Read the model definition and answer for the solid it produces. Units are mm, in the model's axes. A direction names the side the tool comes from. Round coordinates to 2 decimals unless told otherwise and drop trailing zeros. Order: outer loops, then holes, each group sorted by start corner. A loop starts at its lowest first (then second) coordinate and runs counter-clockwise, first axis right, second up. Notation, with made-up numbers: (49.25, 43.5) -> (105.25, 43.5) arc R22 cw to (105.25, 69.5) -> close; hole circle Ø10 at (-8, 77). An arc over 180 degrees is marked (long way). Use a Markdown table: item, result. Add a question column.
1. Section B-B, the plane y = -12.5 is taken. Give the number of separate pieces and of enclosed holes in the cut face, then the cut area to 3 significant figures.
2. For faces 5 (the face through (165.216, -15, -110)), 6 (the face through (-25, -20, -110)), 7 (the face through (100, -15, 265)), 8 (the face through (-4, 0, -4)), determine the directions among +Z, -Z, +X, -X, +Y, -Y from which every point of the face is accessible in a straight line to the end or side of a thin tool.
3. Section A-A, the plane z = 16.5 is taken. Give the vertices of the cut face in (x, y).
4. The mould has two halves that part along X. Classify faces 1 (the face through (-4, -30, -4)), 2 (the face through (-110, -15, -110)), 3 (the face through (-282.89, -14.79, 281.96)), 4 (the face through (65, -10, 120)): +X half, -X half, draft (parallel to the pull), parting line (faces both ways), or undercut.
5. Consider L1, parallel to X at y = -15.75, z = -60; L2, parallel to X at y = -20.5, z = 34.5; L3, parallel to X at y = -17.25, z = 160. Determine where each line is inside the solid, lowest interval first. Write a range as [from, to].
6. Given pin 1 (15 mm diameter, centred on x = -55.5, z = -105, fed in from -Y), flat-ended and moving along its own axis, determine where the tip first touches the part or whether it passes through.
```python
from build123d import *

# Parameters (mm, degrees)
EXTRUDE_1715_DEPTH     = 30
SKETCH_1780_R          = 2.5
CUT_EXTRUDE_1807_DEPTH = 426.323406363
CUT_EXTRUDE_2500_DEPTH = 426.323406363
CUT_EXTRUDE_START      = 10
CUT_EXTRUDE_3097_DEPTH = 10


with BuildPart() as part:
    # Sketch 1708 → Extrude 1715 (new body)
    with BuildSketch(Plane(origin=(0, 0, 0), x_dir=(1, 0, 0), z_dir=(0, 1, 0))):
        with BuildLine():
            Line((-90, -220), (90, -220))
            ThreePointArc((90, -220), (97.071067812, -222.928932188), (100, -230))
            Line((100, -230), (100, -300))
            Line((100, -300), (240, -300))
            ThreePointArc((240, -300), (282.426406871, -282.426406871), (300, -240))
            Line((300, -240), (300, 240))
            ThreePointArc((300, 240), (282.426406871, 282.426406871), (240, 300))
            Line((240, 300), (-240, 300))
            ThreePointArc((-240, 300), (-282.426406871, 282.426406871), (-300, 240))
            Line((-300, 240), (-300, -240))
            ThreePointArc((-300, -240), (-282.426406871, -282.426406871), (-240, -300))
            Line((-240, -300), (-100, -300))
            Line((-100, -300), (-100, -230))
            ThreePointArc((-100, -230), (-97.071067812, -222.928932188), (-90, -220))
        make_face()
    extrude(amount=-EXTRUDE_1715_DEPTH)

    # Sketch 1780 → Cut-Extrude 1807 (cut, through all)
    with BuildSketch(Plane(origin=(0, 0, 0), x_dir=(1, 0, 0), z_dir=(0, 1, 0))):
        with Locations(Location((-115, 60, 0), (0, 0, 270))):
            Circle(SKETCH_1780_R)
        with Locations(Location((47, 60, 0), (0, 0, 270))):
            Circle(SKETCH_1780_R)
        with Locations(Location((210, 60, 0), (0, 0, 270))):
            Circle(SKETCH_1780_R)
        with Locations(Location((-100, -160, 0), (0, 0, 270))):
            Circle(SKETCH_1780_R)
        with Locations(Location((50, -160, 0), (0, 0, 270))):
            Circle(SKETCH_1780_R)
        with Locations(Location((130, -160, 0), (0, 0, 270))):
            Circle(SKETCH_1780_R)
        with Locations(Location((-42.72, 60, 0), (0, 0, 270))):
            Circle(SKETCH_1780_R)
        with Locations(Location((-199.29, 65.75, 0), (0, 0, 270))):
            Circle(SKETCH_1780_R)
        with Locations(Location((-160.19, 185.5, 0), (0, 0, 270))):
            Circle(SKETCH_1780_R)
        with Locations(Location((34.806763, 175.55, 0), (0, 0, 270))):
            Circle(SKETCH_1780_R)
        with Locations(Location((150.216186, 177.55, 0), (0, 0, 270))):
            Circle(SKETCH_1780_R)
        with Locations(Location((212.76, 177.55, 0), (0, 0, 270))):
            Circle(SKETCH_1780_R)
        with Locations(Location((-166.666763, -78.149039, 0), (0, 0, 270))):
            Circle(SKETCH_1780_R)
        with Locations(Location((-219.52, 3.7, 0), (0, 0, 270))):
            Circle(SKETCH_1780_R)
        with Locations(Location((-34.29, -154.25, 0), (0, 0, 270))):
            Circle(SKETCH_1780_R)
        with Locations(Location((4.81, -34.5, 0), (0, 0, 270))):
            Circle(SKETCH_1780_R)
        with Locations(Location((223.895, -100, 0), (0, 0, 270))):
            Circle(SKETCH_1780_R)
        with Locations(Location((130, 10, 0), (0, 0, 270))):
            Circle(SKETCH_1780_R)
    extrude(amount=-CUT_EXTRUDE_1807_DEPTH, mode=Mode.SUBTRACT)

    # Sketch 1847 → Cut-Extrude 2500 (cut, through all)
    with BuildSketch(Plane(origin=(0, 0, 0), x_dir=(1, 0, 0), z_dir=(0, 1, 0))):
        with BuildLine():
            Line((-100, 120), (-100, 100))
            ThreePointArc((-100, 100), (-105, 95), (-110, 100))
            Line((-110, 100), (-110, 120))
            ThreePointArc((-110, 120), (-105, 125), (-100, 120))
        make_face()
        with BuildLine():
            Line((62, 120), (62, 100))
            ThreePointArc((62, 100), (57, 95), (52, 100))
            Line((52, 100), (52, 120))
            ThreePointArc((52, 120), (57, 125), (62, 120))
        make_face()
        with BuildLine():
            Line((165.216186, 120), (165.216186, 100))
            ThreePointArc((165.216186, 100), (160.216186, 95), (155.216186, 100))
            Line((155.216186, 100), (155.216186, 120))
            ThreePointArc((155.216186, 120), (160.216186, 125), (165.216186, 120))
        make_face()
        with BuildLine():
            Line((-151.666763, -110), (-151.666763, -130))
            ThreePointArc((-151.666763, -130), (-156.666763, -135), (-161.666763, -130))
            Line((-161.666763, -130), (-161.666763, -110))
            ThreePointArc((-161.666763, -110), (-156.666763, -105), (-151.666763, -110))
        make_face()
        with BuildLine():
            Line((65, -110), (65, -130))
            ThreePointArc((65, -130), (60, -135), (55, -130))
            Line((55, -130), (55, -110))
            ThreePointArc((55, -110), (60, -105), (65, -110))
        make_face()
        with BuildLine():
            Line((145, -110), (145, -130))
            ThreePointArc((145, -130), (140, -135), (135, -130))
            Line((135, -130), (135, -110))
            ThreePointArc((135, -110), (140, -105), (145, -110))
        make_face()
    extrude(amount=-CUT_EXTRUDE_2500_DEPTH, mode=Mode.SUBTRACT)

    # Sketch 2558 → Cut-Extrude 3097 (cut)
    with BuildSketch(Plane(origin=(0, -30, 0), x_dir=(1, 0, 0), z_dir=(0, 1, 0)).offset(CUT_EXTRUDE_START)):
        with BuildLine():
            Line((-105, 95), (70, 95))
            ThreePointArc((70, 95), (73.535533906, 93.535533906), (75, 90))
            Line((75, 90), (75, -100))
            ThreePointArc((75, -100), (73.535533906, -103.535533906), (70, -105))
            Line((70, -105), (-156.666763, -105))
            ThreePointArc((-156.666763, -105), (-160.202296906, -106.464466094), (-161.666763, -110))
            Line((-161.666763, -110), (-161.666763, -130))
            ThreePointArc((-161.666763, -130), (-160.202296906, -133.535533906), (-156.666763, -135))
            Line((-156.666763, -135), (-10, -135))
            ThreePointArc((-10, -135), (-6.464466094, -136.464466094), (-5, -140))
            Line((-5, -140), (-5, -220))
            Line((-5, -220), (25, -220))
            Line((25, -220), (25, -140))
            ThreePointArc((25, -140), (26.464466094, -136.464466094), (30, -135))
            Line((30, -135), (140, -135))
            ThreePointArc((140, -135), (143.535533906, -133.535533906), (145, -130))
            Line((145, -130), (145, -110))
            ThreePointArc((145, -110), (143.535533906, -106.464466094), (140, -105))
            Line((140, -105), (110, -105))
            ThreePointArc((110, -105), (106.464466094, -103.535533906), (105, -100))
            Line((105, -100), (105, 90))
            ThreePointArc((105, 90), (106.464466094, 93.535533906), (110, 95))
            Line((110, 95), (160.216186, 95))
            ThreePointArc((160.216186, 95), (163.751719906, 96.464466094), (165.216186, 100))
            Line((165.216186, 100), (165.216186, 120))
            ThreePointArc((165.216186, 120), (163.751719906, 123.535533906), (160.216186, 125))
            Line((160.216186, 125), (-105, 125))
            ThreePointArc((-105, 125), (-108.535533906, 123.535533906), (-110, 120))
            Line((-110, 120), (-110, 100))
            ThreePointArc((-110, 100), (-108.535533906, 96.464466094), (-105, 95))
        make_face()
    extrude(amount=-CUT_EXTRUDE_3097_DEPTH, mode=Mode.SUBTRACT)


solid = part.part
```
Verdict:
| question | item | result |
|---|---|---|
| 1 | separate pieces | 1 |
| 1 | enclosed holes | 24 |
| 1 | area | 339,000 mm2 |
| 2 | face 5 | +Y, -Y |
| 2 | face 6 | -Y |
| 2 | face 7 | +Z, +Y, -Y |
| 2 | face 8 | +Z, -Z, +X, -X, +Y |
| 3 | outline | (-300, -30) -> (75, -30) -> (75, -20) -> (105, -20) -> (105, -30) -> (300, -30) -> (300, 0) -> (-300, 0) -> close |
| 4 | face 1 | draft |
| 4 | face 2 | undercut |
| 4 | face 3 | -X half |
| 4 | face 4 | undercut |
| 5 | L1 | x = [-300, -117.5], [-112.5, -45.22], [-40.22, 44.5], [49.5, 207.5], [212.5, 300] |
| 5 | L2 | x = [-300, 2.31], [7.31, 75], [105, 300] |
| 5 | L3 | x = [-300, -102.5], [-97.5, 47.5], [52.5, 127.5], [132.5, 300] |
| 6 | pin 1 | stops at y = -20 |
